Source: CAD feature listing. Evaluate the final solid. Frame: model axes, mm. Face numbers are marked on the shaded views. Coordinates: 2 decimals unless noted, no trailing zeros. Write each loop counter-clockwise with the first axis right and the second up, starting at its lowest first coordinate (ties: lowest second). Pieces come first, ordered by that corner, then holes. Notation, with made-up numbers: M 24,15.25 L 83,15.25 A17 ccw 83,48.25 Z; hole C -31,45.5 d1. An arc over 180 degrees is marked long. Answer as CSV lines item,"result". Start each with the question number.
1. Mould query, pull axis Y, two halves, no side actions, for the marked faces 1, 2 and 3. Classes: pulls with the +Y half, pulls with the -Y half, needs draft (parallel to the pull), parting line crosses it, or undercut.
2. Line query: probe 1 along Y at (x, z) = (207.5, -156); probe 2 along Z at (x, y) = (271, 177.75); probe 3 along Y at (x, z) = (270.5, -156.25). Output: solid intervals per line, ascending. Write a range as [from, to].
3. Contact query for flat-ended pins moving along their axis: pin 1 Ø1.5 at (x, z) = (217, -166.5) entering from -Y; pin 2 Ø1.5 at (x, z) = (257.5, -155.5) entering from +Y; pin 3 Ø2 at (y, z) = (186, -158.5) entering from -X; pin 4 Ø8 at (x, y) = (208.5, 174) entering from -Z. Output: stop coordinate, or through.
4. Section B-B on z = -161.5. Return the cut outline in (x, y).
5. Section A-A on y = 184.5. Return the cut outline in (x, z), plus the area to 3 significant figures.
6. Section C-C on x = 258.5. Return the cut outline in (y, z), plus the area to 3 significant figures.
7. Section D-D on y = 190. Return the cut outline in (x, z), plus the area to 3 significant figures.
```python
from build123d import *

# Parameters (mm, degrees)
BOSS_EXTRUDE1_DEPTH = 121.6025


with BuildPart() as part:
    # Sketch1 → Boss-Extrude1 (new body)
    with BuildSketch(Plane(origin=(193.3575, 0, 0), x_dir=(0, 0, -1), z_dir=(1, 0, 0))):
        with BuildLine():
            ThreePointArc((169.472564712, 184.756731005), (157.228913048, 190.791231973), (151.19441208, 178.547580309))
            ThreePointArc((151.19441208, 178.547580309), (163.438063744, 172.513079341), (169.472564712, 184.756731005))
        make_face()
        Polygon((157.971317168, 188.605783997), (153.130383991, 183.083269536), (155.492555219, 176.129641196), (162.695659624, 174.698527317), (167.536592801, 180.221041778), (165.174421573, 187.174670118), align=None, mode=Mode.SUBTRACT)
    extrude(amount=BOSS_EXTRUDE1_DEPTH)


solid = part.part
```
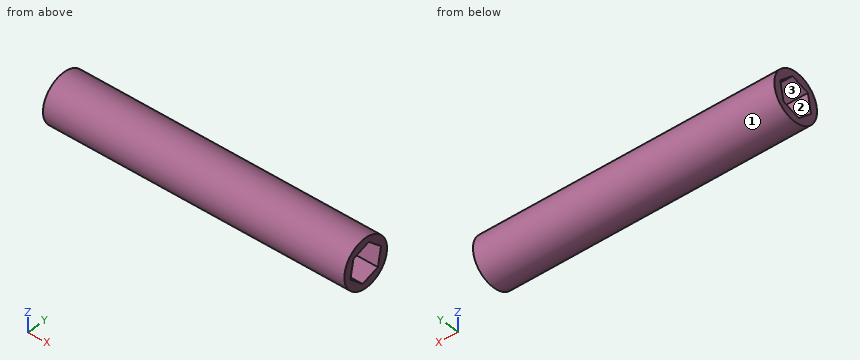
Values:
1,face 1,"parting line crosses it"
1,face 2,"undercut"
1,face 3,"undercut"
2,probe 1,"[173.03, 176.03], [186.36, 190.28]"
2,probe 2,"[-169.16, -165.37], [-154.94, -151.51]"
2,probe 3,"[172.91, 175.98], [186.64, 190.4]"
3,pin 1,"y = 173.66"
3,pin 2,"y = 190.4"
3,pin 3,"through"
3,pin 4,"z = -169.27"
4,outline,"M 193.36,172.07 L 314.96,172.07 L 314.96,174.94 L 193.36,174.94 Z; M 193.36,187.9 L 314.96,187.9 L 314.96,191.23 L 193.36,191.23 Z"
5,outline,"M 193.36,-169.56 L 314.96,-169.56 L 314.96,-166.08 L 193.36,-166.08 Z; M 193.36,-154.37 L 314.96,-154.37 L 314.96,-151.11 L 193.36,-151.11 Z"
5,area,"819 mm²"
6,outline,"C 181.65,-160.33 d19.3; hole M 174.7,-162.7 L 180.22,-167.54 L 187.17,-165.17 L 188.61,-157.97 L 183.08,-153.13 L 176.13,-155.49 Z"
6,area,"153 mm²"
7,outline,"M 193.36,-165.18 L 314.96,-165.18 L 314.96,-155.49 L 193.36,-155.49 Z"
7,area,"1,180 mm²"
